Model file for the job. Use its own axes, mm. Give positions to 0.01 mm unless a question says otherwise; leave off trailing zeros. Loops run counter-clockwise (first coordinate to the right, second up) from the corner with the lowest first, then second, coordinate; pieces in that order, holes last. Notation, with made-up numbers: (26.5, -34.5) - (38.5, -34.5) arc R27 cw to (38.5, -12.5) - close; hole circle Ø8 at (87, 2). An arc over 180 degrees is marked (long way). Use a Markdown table: item, result.
from build123d import *

# Parameters (mm, degrees)
SKETCH_W    = 45
SKETCH_H    = 33.4
PAD_DEPTH   = 143
FILLET_R    = 8
FILLET001_R = 2.5


with BuildPart() as part:
    # Sketch → Pad (new body)
    with BuildSketch(Plane.XY):
        Rectangle(SKETCH_W, SKETCH_H)
    extrude(amount=PAD_DEPTH)

    # Fillet
    fillet_edges = [part.edges().sort_by_distance(p)[0] for p in [
        (22.5, -16.7, 71.5),
        (22.5, 16.7, 71.5),
        (-22.5, -16.7, 71.5),
        (-22.5, 16.7, 71.5),
    ]]
    fillet(fillet_edges, radius=FILLET_R)

    # Fillet001
    fillet001_edges = [part.edges().sort_by_distance(p)[0] for p in [
        (0, -16.7, 143),
        (20.156854, -14.356854, 143),
        (22.5, 0, 143),
        (20.156854, 14.356854, 143),
        (0, 16.7, 143),
        (-20.156854, 14.356854, 143),
        (-22.5, 0, 143),
        (-20.156854, -14.356854, 143),
        (20.156854, -14.356854, 0),
        (0, -16.7, 0),
        (-20.156854, -14.356854, 0),
        (-22.5, 0, 0),
        (-20.156854, 14.356854, 0),
        (0, 16.7, 0),
        (20.156854, 14.356854, 0),
        (22.5, 0, 0),
    ]]
    fillet(fillet001_edges, radius=FILLET001_R)


solid = part.part
(1) Pin check, flat tip, straight feed: P1, Ø3, axis at y = -10.5, z = 31, coming from the +X side. Stop position of the tip, or through.
Computed:
| item | result |
|---|---|
| P1 | x = 22.49 |
(2) Drill centre lines: probe 1 along X at (y, z) = (9, 11); probe 2 along Y at (x, z) = (-17, 53); probe 3 along Y at (x, z) = (20, 59). Where is each one in solid material? Low to high. Write a range as [from, to].
Computed:
| item | result |
|---|---|
| probe 1 | [-22.49, 22.49] |
| probe 2 | [-16.3, 16.3] |
| probe 3 | [-14.51, 14.51] |
(3) Slice it at A-A, the plane z = 60. Write the cut outline in (x, y).
Computed:
| item | result |
|---|---|
| outline | (-22.5, -8.7) arc R8 ccw to (-14.5, -16.7) - (14.5, -16.7) arc R8 ccw to (22.5, -8.7) - (22.5, 8.7) arc R8 ccw to (14.5, 16.7) - (-14.5, 16.7) arc R8 ccw to (-22.5, 8.7) - close |
